```python
from build123d import *

# Parameters (mm, degrees)
SKETCH3_W                                  = 33
SKETCH3_H                                  = 33
BOSS_EXTRUDE1_DEPTH                        = 20
SKETCH4_W                                  = 33
SKETCH4_H                                  = 12
CUT_EXTRUDE1_DEPTH                         = 7
MIRROR7_AT_THE_SECOND_PLANE_COPY_1_SKETC_W = 33
MIRROR7_AT_THE_SECOND_PLANE_COPY_1_SKETC_H = 12
MIRROR7_AT_THE_SECOND_PLANE_COPY_1_DEPTH   = 7
SKETCH6_W                                  = 19
SKETCH6_H                                  = 12
CUT_EXTRUDE2_DEPTH                         = 7
MIRROR8_AT_THE_SECOND_PLANE_COPY_1_SKETC_W = 19
MIRROR8_AT_THE_SECOND_PLANE_COPY_1_SKETC_H = 12
MIRROR8_AT_THE_SECOND_PLANE_COPY_1_DEPTH   = 7
SKETCH7_R                                  = 6
CUT_EXTRUDE3_DEPTH                         = 31.732718721
SKETCH9_R                                  = 1.5
CUT_EXTRUDE5_DEPTH                         = 7.5
SKETCH10_R                                 = 1.5
CUT_EXTRUDE9_DEPTH                         = 4


with BuildPart() as part:
    # Sketch3 → Boss-Extrude1 (new body)
    with BuildSketch(Plane(origin=(0, 0, 0), x_dir=(1, 0, 0), z_dir=(0, 1, 0))):
        Rectangle(SKETCH3_W, SKETCH3_H)
    extrude(amount=BOSS_EXTRUDE1_DEPTH)

    # Sketch4 → Cut-Extrude1 (cut)
    with BuildSketch(Plane.XY.offset(16.5)):
        with Locations((0, 10)):
            Rectangle(SKETCH4_W, SKETCH4_H)
    cut_extrude1 = extrude(amount=-CUT_EXTRUDE1_DEPTH, mode=Mode.SUBTRACT)

    # Mirror7: Cut-Extrude1 across plane
    add(cut_extrude1.mirror(Plane(origin=(0, 0, 0), x_dir=(0, 0, 1), z_dir=(1, 0, 0))), mode=Mode.SUBTRACT)

    # Mirror7 at the second plane: Cut-Extrude1 across plane
    add(cut_extrude1.mirror(Plane.XY), mode=Mode.SUBTRACT)

    # Mirror7 at the second plane copy 1 sketc → Mirror7 at the second plane copy 1 (cut)
    with BuildSketch(Plane(origin=(0, 0, -16.5), x_dir=(-1, 0, 0), z_dir=(0, 0, -1))):
        with Locations((0, 10)):
            Rectangle(MIRROR7_AT_THE_SECOND_PLANE_COPY_1_SKETC_W, MIRROR7_AT_THE_SECOND_PLANE_COPY_1_SKETC_H)
    extrude(amount=-MIRROR7_AT_THE_SECOND_PLANE_COPY_1_DEPTH, mode=Mode.SUBTRACT)

    # Sketch6 → Cut-Extrude2 (cut)
    with BuildSketch(Plane(origin=(16.5, 0, 0), x_dir=(0, 0, -1), z_dir=(1, 0, 0))):
        with Locations((0, 10)):
            Rectangle(SKETCH6_W, SKETCH6_H)
    cut_extrude2 = extrude(amount=-CUT_EXTRUDE2_DEPTH, mode=Mode.SUBTRACT)

    # Mirror8: Cut-Extrude2 across plane
    add(cut_extrude2.mirror(Plane.XY), mode=Mode.SUBTRACT)

    # Mirror8 at the second plane: Cut-Extrude2 across plane
    add(cut_extrude2.mirror(Plane(origin=(0, 0, 0), x_dir=(0, 0, 1), z_dir=(1, 0, 0))), mode=Mode.SUBTRACT)

    # Mirror8 at the second plane copy 1 sketc → Mirror8 at the second plane copy 1 (cut)
    with BuildSketch(Plane.ZY.offset(16.5)):
        with Locations((0, 10)):
            Rectangle(MIRROR8_AT_THE_SECOND_PLANE_COPY_1_SKETC_W, MIRROR8_AT_THE_SECOND_PLANE_COPY_1_SKETC_H)
    extrude(amount=-MIRROR8_AT_THE_SECOND_PLANE_COPY_1_DEPTH, mode=Mode.SUBTRACT)

    # Sketch7 → Cut-Extrude3 (cut, through all)
    with BuildSketch(Plane(origin=(0, 20, 0), x_dir=(1, 0, 0), z_dir=(0, 1, 0))):
        with Locations(Location((0, 0, 0), (0, 0, 270))):
            Circle(SKETCH7_R)
    extrude(amount=-CUT_EXTRUDE3_DEPTH, mode=Mode.SUBTRACT)

    # Sketch9 → Cut-Extrude5 (cut, symmetric)
    with BuildSketch(Plane(origin=(0, 20, 0), x_dir=(1, 0, 0), z_dir=(0, 1, 0))):
        with Locations(Location((0, 12.5, 0), (0, 0, 180))):
            Circle(SKETCH9_R)
    extrude(amount=CUT_EXTRUDE5_DEPTH, both=True, mode=Mode.SUBTRACT)

    # Sketch10 → Cut-Extrude9 (cut, symmetric)
    with BuildSketch(Plane.XY.offset(9.5)):
        with Locations(Location((0, 8, 0), (0, 0, 90))):
            Circle(SKETCH10_R)
    extrude(amount=CUT_EXTRUDE9_DEPTH, both=True, mode=Mode.SUBTRACT)


solid = part.part
```
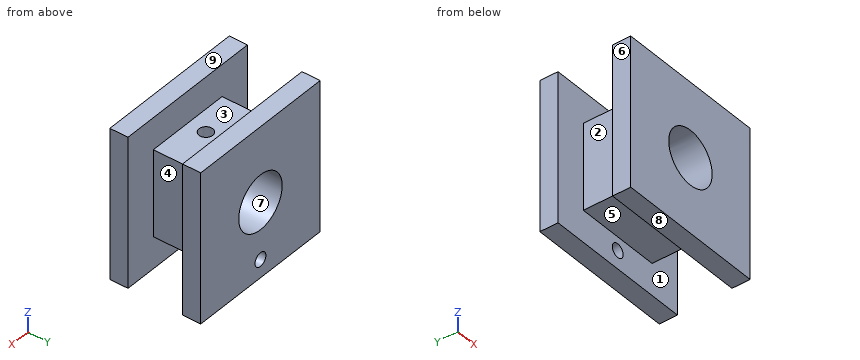
Geometry: final body of the model. Coordinates: model frame, mm. Face numbers are marked on the shaded views. A direction names the side the tool comes from. Give positions to 0.01 mm unless a question says otherwise; leave off trailing zeros. Loops run counter-clockwise (first coordinate to the right, second up) from the corner with the lowest first, then second, coordinate; pieces in that order, holes last. Notation, with made-up numbers: (-33.5, 47) - (1.5, 47) arc R24 ccw to (1.5, 86) - close; hole circle Ø7 at (53, 3). An arc over 180 degrees is marked (long way). Answer as CSV lines item,"result". Start each with the question number.
(1) Section query A-A (x = -14). Output: boundary loops of the cut face in (y, z).
(2) Reachability of the marked faces 1, 2, 3, 4 and 5 from +Z, -Z, +X, -X, +Y, -Y: full face, straight path, thin tool, end or side. Return the list, or none.
(3) Pin query (flat end, axial travel): P1, Ø1.8, axis at x = 0, y = 8, coming from the -Z side; P2, Ø3.5, axis at y = 9, z = -1, coming from the +X side; P3, Ø3.5, axis at x = 0.5, y = 9.5, coming from the +Z side; P4, Ø9.5, axis at x = 0, z = 0, coming from the -Y side (1 decimal). Return the tip coordinate at first contact, or that it passes through.
(4) Mould query, pull axis Z, two halves, no side actions, for the marked faces 6, 7, 8 and 9. Classes: +Z half, -Z half, draft (parallel to the pull), parting line (faces both ways), or undercut.
(5) Ray query, line 1 along Y through (x, z) = (7.5, 10); line 2 along X through (y, z) = (8, 7.4); line 3 along X through (y, z) = (6.5, 0). Return the intervals inside material, ascending. Write a range as [from, to].
(6) Section query B-B (z = 0). Output: boundary loops of the cut face in (x, y), and give its area (3 significant figures).
(7) Section query D-D (x = 0). Output: boundary loops of the cut face in (y, z), and give its area (4 significant figures).
(8) Section query C-C (y = 8). Output: boundary loops of the cut face in (x, z).
Worked answers:
1,outline,"(0, -16.5) - (4, -16.5) - (4, 16.5) - (0, 16.5) - close; (16, -16.5) - (20, -16.5) - (20, 16.5) - (16, 16.5) - close"
2,face 1,"none"
2,face 2,"+Z, -Z, -X"
2,face 3,"+Z, +X, -X"
2,face 4,"+Z, -Z, +X"
2,face 5,"-Z, +X, -X"
3,P1,"stops at z = -9.5"
3,P2,"stops at x = 9.5"
3,P3,"stops at z = 9.5"
3,P4,"passes through"
4,face 6,"draft"
4,face 7,"undercut"
4,face 8,"-Z half"
4,face 9,"+Z half"
5,line 1,"y = [0, 4], [16, 20]"
5,line 2,"x = [-9.5, -1.5], [1.5, 9.5]"
5,line 3,"x = [-9.5, -6], [6, 9.5]"
6,outline,"(-16.5, 0) - (-6, 0) - (-6, 20) - (-16.5, 20) - (-16.5, 16) - (-9.5, 16) - (-9.5, 4) - (-16.5, 4) - close; (6, 0) - (16.5, 0) - (16.5, 4) - (9.5, 4) - (9.5, 16) - (16.5, 16) - (16.5, 20) - (6, 20) - close"
6,area,"252 mm^2"
7,outline,"(0, -16.5) - (4, -16.5) - (4, -9.5) - (16, -9.5) - (16, -11) - (20, -11) - (20, -6) - (0, -6) - close; (0, 6) - (6.5, 6) - (6.5, 9.5) - (4, 9.5) - (4, 16.5) - (0, 16.5) - close; (9.5, 6) - (20, 6) - (20, 16.5) - (16, 16.5) - (16, 9.5) - (9.5, 9.5) - close; (16, -16.5) - (20, -16.5) - (20, -14) - (16, -14) - close"
7,area,"229.5 mm^2"
8,outline,"(-9.5, -9.5) - (9.5, -9.5) - (9.5, 9.5) - (1.5, 9.5) - (1.5, 5.81) arc R6 cw (long way) to (-1.5, 5.81) - (-1.5, 9.5) - (-9.5, 9.5) - close"
